The model under review builds one solid part; all positions refer to its coordinate system, in mm. A direction names the side the tool comes from. Round coordinates to 2 decimals unless told otherwise and drop trailing zeros. Loops run counter-clockwise (first coordinate to the right, second up) from the corner with the lowest first, then second, coordinate; pieces in that order, holes last. Notation, with made-up numbers: M 87,45.25 L 133,45.25 A19 ccw 133,49.25 Z; hole C -38,27 d1. An arc over 180 degrees is marked long. One line per question, with ' | ' between items.
from build123d import *

# Parameters (mm, degrees)
SKETCH1_W           = 35.56
SKETCH1_H           = 35.56
BOSS_EXTRUDE1_DEPTH = 34
SKETCH2_R           = 2.5
BOSS_EXTRUDE2_DEPTH = 24
SKETCH3_R           = 2.5
BOSS_EXTRUDE3_DEPTH = 12
SKETCH4_R           = 2
CUT_EXTRUDE1_DEPTH  = 34


with BuildPart() as part:
    # Sketch1 → Boss-Extrude1 (new body)
    with BuildSketch(Plane(origin=(0, 0, 0), x_dir=(1, 0, 0), z_dir=(0, 1, 0))):
        Rectangle(SKETCH1_W, SKETCH1_H)
    extrude(amount=BOSS_EXTRUDE1_DEPTH)

    # Sketch2 → Boss-Extrude2 (add)
    with BuildSketch(Plane(origin=(0, 34, 0), x_dir=(1, 0, 0), z_dir=(0, 1, 0))):
        Circle(SKETCH2_R)
    extrude(amount=BOSS_EXTRUDE2_DEPTH)

    # Sketch3 → Boss-Extrude3 (add)
    with BuildSketch(Plane.XZ):
        Circle(SKETCH3_R)
    extrude(amount=BOSS_EXTRUDE3_DEPTH)

    # Sketch4 → Cut-Extrude1 (cut)
    with BuildSketch(Plane(origin=(0, 34, 0), x_dir=(1, 0, 0), z_dir=(0, 1, 0))):
        with Locations((-13, 13)):
            Circle(SKETCH4_R)
        with Locations((13, 13)):
            Circle(SKETCH4_R)
        with Locations((13, -13)):
            Circle(SKETCH4_R)
        with Locations((-13, -13)):
            Circle(SKETCH4_R)
    extrude(amount=-CUT_EXTRUDE1_DEPTH, mode=Mode.SUBTRACT)


solid = part.part
1) Add section B-B on x = -1.5. State the section outline as (y, z) points, then the cut area to 3 significant figures.
Output values:
outline: M -12,-2 L 0,-2 L 0,-17.78 L 34,-17.78 L 34,-2 L 58,-2 L 58,2 L 34,2 L 34,17.78 L 0,17.78 L 0,2 L -12,2 Z | area: 1,350 mm²
2) Add section A-A on z = 13. State the section outline as (x, y) points.
Output values:
outline: M -17.78,0 L -15,0 L -15,34 L -17.78,34 Z; M -11,0 L 11,0 L 11,34 L -11,34 Z; M 15,0 L 17.78,0 L 17.78,34 L 15,34 Z
3) Machinability: for faces 1 (the cylindrical face through (-0.54, 45.83, 2.44)), 2 (the flat face through (17.78, 17, 0)), which of the approach directions +Z, -Z, +X, -X, +Y, -Y give a long, thin tool a straight path to every point of the face, cutting with its end or side? Answer none if there is none.
Output values:
face 1: +Y | face 2: +Z, -Z, +X, +Y, -Y
4) Insertion check: P1, Ø3, axis at x = -13, z = -13, coming from the +Y side; P2, Ø5, axis at x = -13, z = 13, coming from the +Y side; P3, Ø4, axis at x = 3.5, z = 4.5, coming from the -Y side. Each pin has a flat end and moves straight along its axis. Give the tip position at first contact, or say it passes through.
Output values:
P1: passes through | P2: stops at y = 34 | P3: stops at y = 0
5) Add section D-D on x = 13. State the section outline as (y, z) points, then the cut area to 3 significant figures.
Output values:
outline: M 0,-17.78 L 34,-17.78 L 34,-15 L 0,-15 Z; M 0,-11 L 34,-11 L 34,11 L 0,11 Z; M 0,15 L 34,15 L 34,17.78 L 0,17.78 Z | area: 937 mm²
6) For line 1 (X direction, y = 19, z = -13); line 2 (Z direction, x = 0, y = 50), list the stretches that pass through material, from the lowest coordinate up.
Output values:
line 1: x = -17.78 to -15, -11 to 11, 15 to 17.78 | line 2: z = -2.5 to 2.5
7) Mouldability with a two-part tool opening along Z and no side actions: class faces 3 (the flat face through (0, 17, 17.78)), 4 (the cylindrical face through (11.526, 17.238, -14.352)), 5 (the cylindrical face through (-0.54, -5.92, -2.44)), 6 (the cylindrical face through (-14.474, 17.238, 11.648)) as +Z half, -Z half, draft (parallel to the pull), parting line (faces both ways), or undercut.
Output values:
face 3: +Z half | face 4: undercut | face 5: parting line | face 6: undercut
8) Add section C-C on y = 9. State the section outline as (x, z) points, then the cut area to 3 significant figures.
Output values:
outline: M -17.78,-17.78 L 17.78,-17.78 L 17.78,17.78 L -17.78,17.78 Z; hole C -13,-13 d4; hole C -13,13 d4; hole C 13,-13 d4; hole C 13,13 d4 | area: 1,210 mm²
